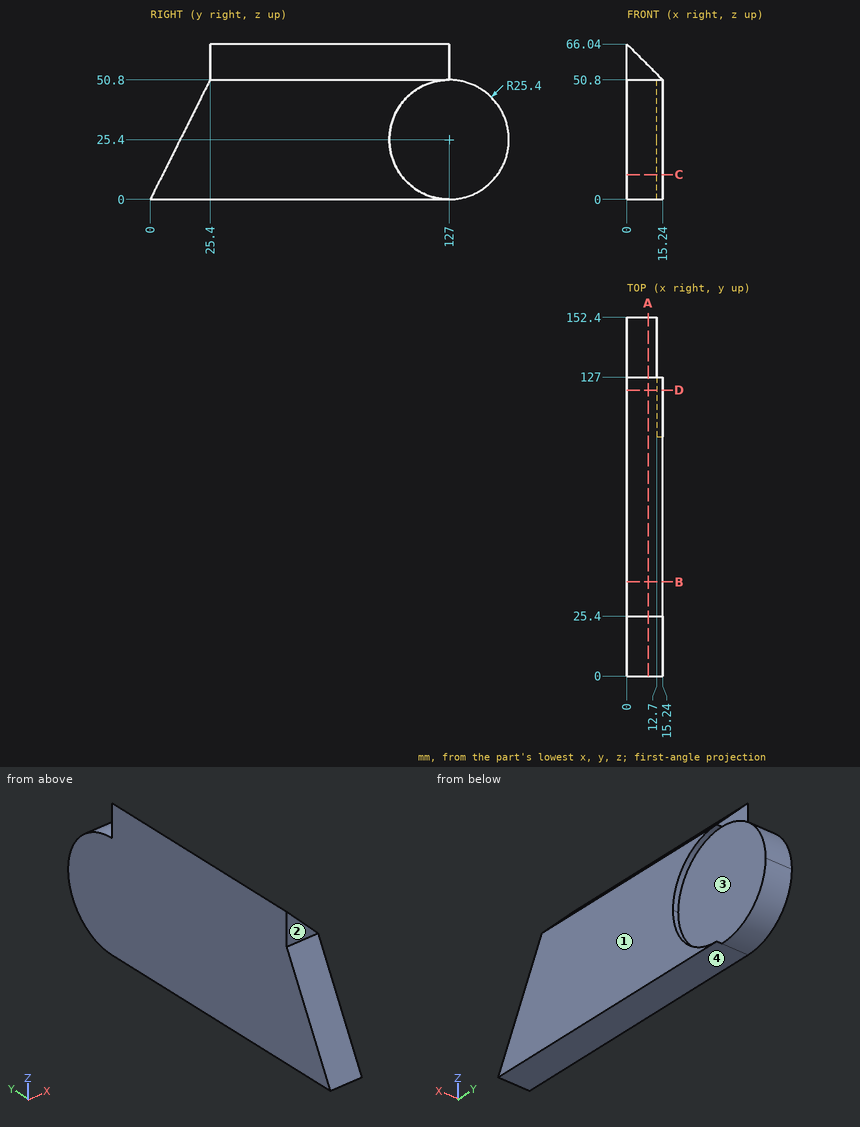
Source: three-view drawing plus pictorial views. Frame: mm from the lowest corner of the part. A direction names the side the tool comes from. Round coordinates to 2 decimals unless told otherwise and drop trailing zeros. Write each loop counter-clockwise with the first axis right and the second up, starting at its lowest first coordinate (ties: lowest second). Pieces come first, ordered by that corner, then holes. Notation, with made-up numbers: M 53.5,8.5 L 106.5,8.5 A27 cw 106.5,39.5 Z; hole C 44.25,-12.75 d2. An arc over 180 degrees is marked long. One line per item, written item: value. Start each with the question number.
Item 1: Section query A-A (x = 9). Return the cut outline in (y, z).
Item 2: Section query B-B (y = 40). Return the cut outline in (x, z).
Item 3: Ray query, L1, parallel to X at y = 131, z = 24.5; L2, parallel to Y at x = 10.5, z = 54; L3, parallel to Z at x = 5.5, y = 80. Return the intervals inside material, ascending. Write a range as from..to.
Item 4: Section query D-D (y = 121.5). Return the cut outline in (x, z), plus the area to 3 significant figures.
Item 5: Pin query (flat end, axial travel): pin 1 (4 mm diameter, centred on x = 13, z = 52, fed in from -Y); pin 2 (7.5 mm diameter, centred on x = 10, z = 59, fed in from -Y); pin 3 (1 mm diameter, centred on x = 3, z = 32.5, fed in from +Y). Return the tip coordinate at first contact, or that it passes through.
Item 6: Set-up query: the marked faces 3 and 4. Return all of +Z, -Z, +X, -X, +Y, -Y with unobstructed straight access to the full face (end or side cutting, diameter ignored); none if empty.
Item 7: Mould query, pull axis Y, two halves, no side actions, for the marked faces 1 and 2. Classes: pulls with the +Y half, pulls with the -Y half, needs draft (parallel to the pull), parting line crosses it, or undercut.
Item 8: Section query C-C (z = 10.5). Return the cut outline in (x, y), plus the area to 3 significant figures.
Result set:
1. outline: M 0,0 L 127,0 A25.4 ccw 127,50.8 L 127,57.04 L 25.4,57.04 L 25.4,50.8 Z
2. outline: M 0,0 L 15.24,0 L 15.24,50.8 L 0,66.04 Z
3. L1: x = 0..12.7
3. L2: y = 25.4..127
3. L3: z = 0..60.54
4. outline: M 0,0 L 15.24,0 L 15.24,0.6 L 12.7,0.6 L 12.7,50.2 L 15.24,50.2 L 15.24,50.8 L 0,66.04 Z
4. area: 764 mm²
5. pin 1: stops at y = 25
5. pin 2: stops at y = 25.4
5. pin 3: stops at y = 151.53
6. face 3: +X, +Y
6. face 4: -Z, +X, -X, +Y, -Y
7. face 1: needs draft
7. face 2: pulls with the -Y half
8. outline: M 0,5.25 L 15.24,5.25 L 15.24,106.43 L 12.7,106.43 L 12.7,147.57 L 0,147.57 Z
8. area: 2,060 mm²
